Verification items for the finished model (mm, model axes). Face numbers are marked on the shaded views. A direction names the side the tool comes from. Coordinates: 2 decimals unless noted, no trailing zeros. Order: outer loops, then holes, each group sorted by start corner. A loop starts at its lowest first (then second) coordinate and runs counter-clockwise, first axis right, second up. Notation, with made-up numbers: (-2, 8.25) - (34, 8.25) arc R9 ccw to (34, 16.25) - close; hole circle Ø1 at (-22.5, 44.5). An arc over 180 degrees is marked (long way). Answer as CSV lines item,"result". Start each with the question number.
1. Set-up check for the marked faces 1, 2 and 3: record each of +Z, -Z, +X, -X, +Y, -Y from which the full face is reachable in a straight line by a thin tool's end or side.
2. Section check A-A (y = 0). Record the cut outline in (x, z), and give its area (3 significant figures).
3. Go/stop test with flat-tipped pins: pin 1 (6 mm diameter, centred on x = -116, y = -7, fed in from -Z); pin 2 (3 mm diameter, centred on x = -19.5, z = -28, fed in from +Y); pin 3 (4 mm diameter, centred on y = 7, z = -3, fed in from +X). Record where each tip stops, or that it passes through.
4. Section check B-B (x = -49). Record the cut outline in (y, z).
5. Material ranges on L1, parallel to Z at x = -104, y = 0.5; L2, parallel to Y at x = -38, z = -30; L3, parallel to X at y = 0, z = 1.35, recorded low to high. Write a range as [from, to].
from build123d import *

# Parameters (mm, degrees)
F1_R     = 23.1230345184
F1_R_2   = 19.55
F3_DEPTH = 5
F4_DEPTH = 42


with BuildPart() as f2:
    # F2: sweep along a path in F0
    with BuildLine(Plane.XZ) as f2_path:
        Line((23.1230345184, 0), (23.1230345184, -18.8757088035))
        Line((23.1230345184, -18.8757088035), (-2.4573525631, -29.9991816282))
        Line((-2.4573525631, -29.9991816282), (-99.7967123985, -29.9991816282))
    # F1 (on Top) → F2 (sweep)
    with BuildSketch(Plane.XY):
        with Locations((23.1230345184, 0)):
            Circle(F1_R)
        with Locations((23.1230345184, 0)):
            Circle(F1_R_2, mode=Mode.SUBTRACT)
    sweep(path=f2_path.line, transition=Transition.RIGHT)

    # F1 (on Top) → F3 (join)
    with BuildSketch(Plane.XY):
        with Locations((23.1230345184, 0)):
            Circle(F1_R)
        with Locations((23.1230345184, 0)):
            Circle(F1_R_2, mode=Mode.SUBTRACT)
    extrude(amount=F3_DEPTH)

    # F4 (add): a face of the model
    f4_faces = [f2.faces().sort_by_distance(p)[0] for p in [
        (-99.7967123985, 0, -7.5301652902),
    ]]
    extrude(f4_faces, amount=F4_DEPTH)


solid = f2.part
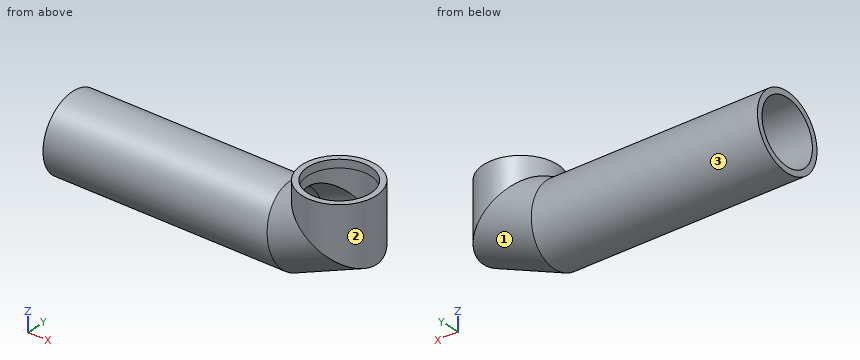
Evaluation:
1,face 1,"none"
1,face 2,"+Z"
1,face 3,"-X"
2,outline,"(-141.8, -53.12) - (2.35, -53.12) - (46.25, -34.04) - (46.25, 5) - (42.67, 5) - (42.67, -31.69) - (1.61, -49.55) - (-141.8, -49.55) - close; (-141.8, -10.45) - (-6.52, -10.45) - (3.57, -6.06) - (3.57, 5) - (0, 5) - (0, -3.72) - (-7.27, -6.88) - (-141.8, -6.88) - close"
2,area,"1,370 mm²"
3,pin 1,"stops at z = -52.77"
3,pin 2,"stops at y = 23.12"
3,pin 3,"stops at x = 45.7"
4,outline,"circle Ø46.25 at (0, -30); hole circle Ø39.1 at (0, -30)"
5,L1,"z = [-53.12, -49.54], [-10.46, -6.88]"
5,L2,"y = [-23.12, -19.55], [19.55, 23.12]"
5,L3,"x = [0, 3.57], [42.67, 46.25]"
